from build123d import *

# Parameters (mm, degrees)
SKETCH1_W           = 51
SKETCH1_H           = 43
SKETCH1_R           = 4.5
SKETCH1_R_2         = 1
SKETCH1_R_3         = 2
SKETCH1_R_4         = 0.5
BOSS_EXTRUDE1_DEPTH = 2.5
FILLET1_R           = 1
BOSS_EXTRUDE2_DEPTH = 30
CUT_EXTRUDE1_DEPTH  = 67


with BuildPart() as part:
    # Sketch1 → Boss-Extrude1 (new body)
    with BuildSketch(Plane(origin=(0, 0, 0), x_dir=(1, 0, 0), z_dir=(0, 1, 0))):
        Rectangle(SKETCH1_W, SKETCH1_H)
        with Locations(Location((0, 0, 0), (0, 0, 270))):
            Circle(SKETCH1_R, mode=Mode.SUBTRACT)
        with Locations(Location((9.7, 0, 0), (0, 0, 270))):
            Circle(SKETCH1_R_2, mode=Mode.SUBTRACT)
        with Locations(Location((-9.7, 0, 0), (0, 0, 270))):
            Circle(SKETCH1_R_2, mode=Mode.SUBTRACT)
        with Locations(Location((0, 8, 0), (0, 0, 270))):
            Circle(SKETCH1_R_2, mode=Mode.SUBTRACT)
        with Locations(Location((0, -8, 0), (0, 0, 270))):
            Circle(SKETCH1_R_2, mode=Mode.SUBTRACT)
        with Locations(Location((-10, 17.5, 0), (0, 0, 270))):
            Circle(SKETCH1_R_3, mode=Mode.SUBTRACT)
        with Locations(Location((10, 17.5, 0), (0, 0, 270))):
            Circle(SKETCH1_R_3, mode=Mode.SUBTRACT)
        with Locations(Location((-15, 0, 0), (0, 0, 270))):
            Circle(SKETCH1_R_4, mode=Mode.SUBTRACT)
        with Locations(Location((15, 0, 0), (0, 0, 270))):
            Circle(SKETCH1_R_4, mode=Mode.SUBTRACT)
        with Locations(Location((0, -17.375333522, 0), (0, 0, 270))):
            Circle(SKETCH1_R_4, mode=Mode.SUBTRACT)
        with Locations(Location((0, 15.103719109, 0), (0, 0, 270))):
            Circle(SKETCH1_R_4, mode=Mode.SUBTRACT)
        with Locations(Location((6.5, 8, 0), (0, 0, 270))):
            Circle(SKETCH1_R_4, mode=Mode.SUBTRACT)
        with Locations(Location((-6.5, 8, 0), (0, 0, 270))):
            Circle(SKETCH1_R_4, mode=Mode.SUBTRACT)
        with Locations(Location((-6.5, -8, 0), (0, 0, 270))):
            Circle(SKETCH1_R_4, mode=Mode.SUBTRACT)
        with Locations(Location((6.5, -8, 0), (0, 0, 270))):
            Circle(SKETCH1_R_4, mode=Mode.SUBTRACT)
        with BuildLine():
            Line((-20.5, -18.5), (-14.5, -18.5))
            ThreePointArc((-14.5, -18.5), (-13.085786438, -17.914213562), (-12.5, -16.5))
            Line((-12.5, -16.5), (-12.5, -10.5))
            ThreePointArc((-12.5, -10.5), (-13.085786438, -9.085786438), (-14.5, -8.5))
            Line((-14.5, -8.5), (-20.5, -8.5))
            ThreePointArc((-20.5, -8.5), (-21.914213562, -9.085786438), (-22.5, -10.5))
            Line((-22.5, -10.5), (-22.5, -16.5))
            ThreePointArc((-22.5, -16.5), (-21.914213562, -17.914213562), (-20.5, -18.5))
        make_face(mode=Mode.SUBTRACT)
    extrude(amount=BOSS_EXTRUDE1_DEPTH)

    # Fillet1
    fillet1_edges = [part.edges().sort_by_distance(p)[0] for p in [
        (25.5, 1.25, -21.5),
        (25.5, 1.25, 21.5),
        (-25.5, 1.25, 21.5),
        (-25.5, 1.25, -21.5),
    ]]
    fillet(fillet1_edges, radius=FILLET1_R)

    # Sketch2 → Boss-Extrude2 (add)
    with BuildSketch(Plane.XZ):
        with BuildLine():
            Line((-23.5, -21.5), (-23.5, 18.5))
            ThreePointArc((-23.5, 18.5), (-23.207106781, 19.207106781), (-22.5, 19.5))
            Line((-22.5, 19.5), (22.5, 19.5))
            ThreePointArc((22.5, 19.5), (23.207106781, 19.207106781), (23.5, 18.5))
            Line((23.5, 18.5), (23.5, -21.5))
            Line((23.5, -21.5), (24.5, -21.5))
            ThreePointArc((24.5, -21.5), (25.207106781, -21.207106781), (25.5, -20.5))
            Line((25.5, -20.5), (25.5, 20.5))
            ThreePointArc((25.5, 20.5), (25.207106781, 21.207106781), (24.5, 21.5))
            Line((24.5, 21.5), (-24.5, 21.5))
            ThreePointArc((-24.5, 21.5), (-25.207106781, 21.207106781), (-25.5, 20.5))
            Line((-25.5, 20.5), (-25.5, -20.5))
            ThreePointArc((-25.5, -20.5), (-25.207106781, -21.207106781), (-24.5, -21.5))
            Line((-24.5, -21.5), (-23.5, -21.5))
        make_face()
    extrude(amount=BOSS_EXTRUDE2_DEPTH)

    # Sketch3 → Cut-Extrude1 (cut)
    with BuildSketch(Plane(origin=(25.5, 0, 0), x_dir=(0, 0, -1), z_dir=(1, 0, 0))):
        with BuildLine():
            add(Edge.make_bspline(
                [(-20.5, -30), (-5.501277344, -7.754009084), (20.5, -0.280836845)],
                knots=[0, 0, 0, 0.981207698, 0.981207698, 0.981207698], degree=2))
            Line((-20.5, -30), (20.5, -30))
            Line((20.5, -30), (20.5, -0.280836845))
        make_face()
        with BuildLine():
            Line((20.5, -30), (-20.5, -30))
            Line((-20.5, -30), (-11.71480256, -35.881315146))
            Line((-11.71480256, -35.881315146), (34.782094199, -34.613217961))
            Line((34.782094199, -34.613217961), (27.415053414, -3.212716254))
            Line((27.415053414, -3.212716254), (21.5, 0))
            add(Edge.make_bspline(
                [(20.5, -0.280836845), (20.997982091, -0.137709033), (21.5, 0)],
                knots=[0.981207698, 0.981207698, 0.981207698, 1, 1, 1], degree=2))
            Line((20.5, -0.280836845), (20.5, -30))
        make_face()
    extrude(amount=-CUT_EXTRUDE1_DEPTH, mode=Mode.SUBTRACT)


solid = part.part
The model under review builds one solid part; all positions refer to its coordinate system, in mm. A direction names the side the tool comes from. Round coordinates to 2 decimals unless told otherwise and drop trailing zeros. Use CSV: the item, a comma, the result in double quotes.
(1) The part is to be moulded in two halves that separate along X. For faces 4 (the cylindrical face through (-21.9, 1.23, 9.07)), 5 (the flat face through (-18, 1, 18.5)), 6 (the flat face through (0, 1, -21.5)), say which applies: pulls with the +X half, pulls with the -X half, needs draft (parallel to the pull), parting line crosses it, or undercut.
Working result:
face 4,"undercut"
face 5,"undercut"
face 6,"needs draft"
(2) Clearance check with flat-ended pins moving along their axes: P1, Ø4, axis at x = 16.5, y = -10, coming from the -Z side; P2, Ø1.2, axis at x = 0, z = -8, coming from the +Y side; P3, Ø12, axis at x = 17, y = -24.5, coming from the -Z side; P4, Ø14.5, axis at x = 0, z = 0, coming from the -Y side. State where each tip first meets the part, or that it passes through.
Working result:
P1,"stops at z = 19.5"
P2,"passes through"
P3,"stops at z = 19.37"
P4,"stops at y = 0"
(3) Take a section at A-A, the plane z = -16.5. State how many separate pieces and enclosed holes the cut face has, plus the area to 3 significant figures.
Working result:
separate pieces,"3"
enclosed holes,"0"
area,"116 mm^2"
(4) Machinability: for faces 1 (the flat face through (-12.5, 1, 14)), 2 (the flat face through (23.5, -7, 8)), 3 (the flat face through (0, 2.5, -5)), which of the approach directions +Z, -Z, +X, -X, +Y, -Y give a long, thin tool a straight path to every point of the face, cutting with its end or side? Answer none if there is none.
Working result:
face 1,"+Y, -Y"
face 2,"-Z, -Y"
face 3,"+Z, -Z, +X, -X, +Y"
(5) For line 1 (X direction, y = 1.55, z = -8); line 2 (X direction, y = 1.45, z = 0); line 3 (X direction, y = -9, z = 13), list the stretches that pass through material, from the lowest coordinate up.
Working result:
line 1,"x = -25.5 to -7, -6 to -1, 1 to 6, 7 to 25.5"
line 2,"x = -25.5 to -15.5, -14.5 to -10.7, -8.7 to -4.5, 4.5 to 8.7, 10.7 to 14.5, 15.5 to 25.5"
line 3,"x = -25.5 to -23.5, 23.5 to 25.5"
